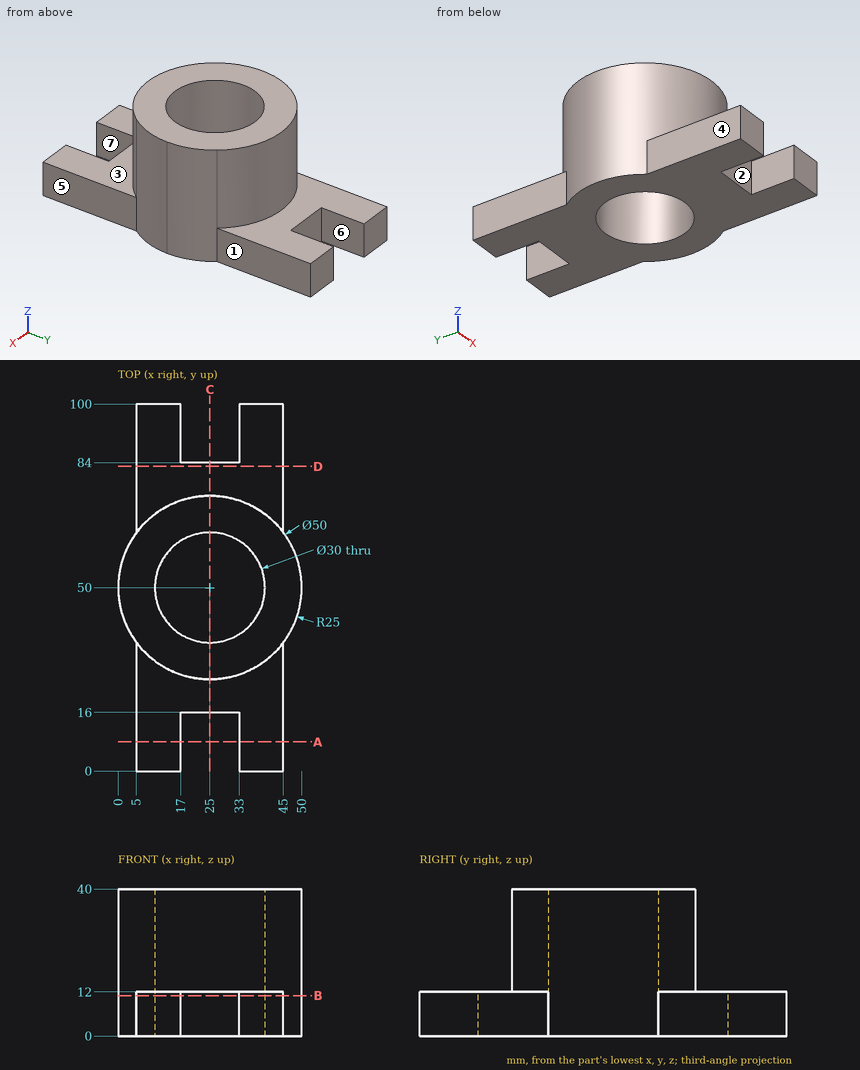
Here's the drawing with two shaded views (mm, measured from the low corner). I have some questions. A direction names the side the tool comes from. Give positions to 0.01 mm unless a question says otherwise; leave off trailing zeros. Write each loop counter-clockwise with the first axis right and the second up, starting at its lowest first coordinate (ties: lowest second). Pieces come first, ordered by that corner, then holes. Notation, with made-up numbers: (33.25, 51.5) -> (40.25, 51.5) arc R15 ccw to (40.25, 74.5) -> close; hole circle Ø3 at (74, 0). An arc over 180 degrees is marked (long way). Use one line per item in the form item = value. Start each with the question number.
1. If I drill on L1, parallel to Y at x = 25, z = 25; L2, parallel to Y at x = 25, z = 9; L3, parallel to X at y = 31, z = 3, over which ranges is the centre line in solid material (lowest first)?
2. Thinking about a two-plate mould opening in X: for the marked faces 1, 2 and 3, which applies, +X half, -X half, draft (parallel to the pull), parting line (faces both ways), or undercut?
3. Imagine slicing it at C-C on x = 25. List the corners of the cut face in (y, z) for me, plus the area to 3 significant figures.
4. Will these pins go through, and if not, where does the flat tip stop? pin 1 Ø2 at (x, z) = (26, 23) entering from +Y; pin 2 Ø13 at (y, z) = (16.5, 7) entering from +X; pin 3 Ø10 at (x, y) = (45, 23) entering from +Z; pin 4 Ø24 at (x, y) = (25, 50) entering from +Z.
5. Imagine slicing it at B-B on z = 11. List the corners of the cut face in (x, y) for me.
6. Imagine slicing it at A-A on y = 8. List the corners of the cut face in (x, z) for me.
7. On a 3-axis mill with a long thin cutter (end or side, diameter ignored), from which of +Z, -Z, +X, -X, +Y, -Y can I reach the whole of each face in a straight line? I mean the marked faces 4, 5, 6 and 7. Say none if no direction works.
8. Imagine slicing it at D-D on y = 83. List the corners of the cut face in (x, z) for me, plus the area to 3 significant figures.
Entries:
q1.L1 = 25 to 35, 65 to 75
q1.L2 = 16 to 35, 65 to 84
q1.L3 = 5 to 45
q2.face_1 = +X half
q2.face_2 = undercut
q2.face_3 = draft
q3.outline = (16, 0) -> (35, 0) -> (35, 40) -> (25, 40) -> (25, 12) -> (16, 12) -> close; (65, 0) -> (84, 0) -> (84, 12) -> (75, 12) -> (75, 40) -> (65, 40) -> close
q3.area = 1,020 mm²
q4.pin_1 = 75
q4.pin_2 = 45
q4.pin_3 = 12
q4.pin_4 = through
q5.outline = (5, 0) -> (17, 0) -> (17, 16) -> (33, 16) -> (33, 0) -> (45, 0) -> (45, 35) arc R25 ccw to (50, 50) arc R25 ccw to (45, 65) -> (45, 100) -> (33, 100) -> (33, 84) -> (17, 84) -> (17, 100) -> (5, 100) -> (5, 65) arc R25 ccw to (5, 35) -> close; hole circle Ø30 at (25, 50)
q6.outline = (5, 0) -> (17, 0) -> (17, 12) -> (5, 12) -> close; (33, 0) -> (45, 0) -> (45, 12) -> (33, 12) -> close
q7.face_4 = +Z, -Z, -X, -Y
q7.face_5 = +Z, -Z, +X, -Y
q7.face_6 = +Z, -Z, +Y
q7.face_7 = +Z, -Z, -Y
q8.outline = (5, 0) -> (45, 0) -> (45, 12) -> (5, 12) -> close
q8.area = 480 mm²
